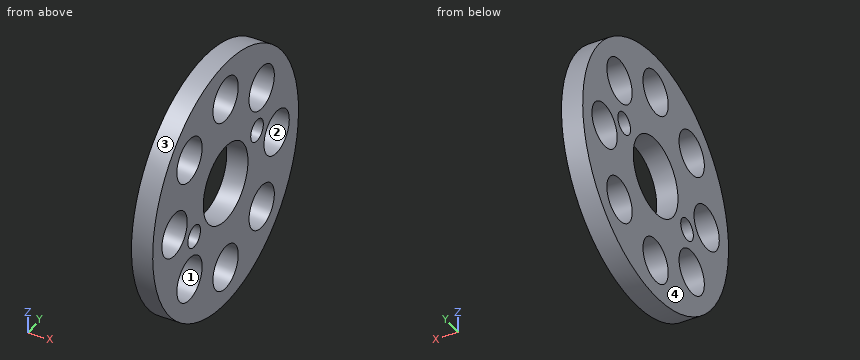
```python
from build123d import *

# Parameters (mm, degrees)
AXIAL_PROFILE_MM_W     = 5
AXIAL_PROFILE_MM_H     = 20.8
AXIAL_HOLES_DEPTH      = 155.634051877
AXIAL_HOLES_DEPTH_BACK = 155.634051877
SKETCH2_R              = 5.2
SKETCH2_R_2            = 2.6


with BuildPart() as part:
    # Axial profile (mm) → Full revolution (revolve)
    with BuildSketch(Plane.XY, mode=Mode.PRIVATE) as full_revolution_sk:
        with Locations((146.2, 19.6)):
            Rectangle(AXIAL_PROFILE_MM_W, AXIAL_PROFILE_MM_H)
    revolve(full_revolution_sk.sketch.rotate(Axis((-110, 0, 0), (1, 0, 0)), 90), axis=Axis((-110, 0, 0), (1, 0, 0)))

    # Sketch2 → Axial holes (cut, two sides: drawn at the far end of the back side and taken through both)
    with BuildSketch(Plane(origin=(0, 0, 0), x_dir=(0, 0, -1), z_dir=(1, 0, 0)).offset(-AXIAL_HOLES_DEPTH_BACK)):
        with Locations((0, 21)):
            Circle(SKETCH2_R)
        with Locations((-14.849242405, 14.849242405)):
            Circle(SKETCH2_R)
        with Locations((-21, 0)):
            Circle(SKETCH2_R)
        with Locations((-14.849242405, -14.849242405)):
            Circle(SKETCH2_R)
        with Locations((0, -21)):
            Circle(SKETCH2_R)
        with Locations((14.849242405, -14.849242405)):
            Circle(SKETCH2_R)
        with Locations((21, 0)):
            Circle(SKETCH2_R)
        with Locations((14.849242405, 14.849242405)):
            Circle(SKETCH2_R)
        with Locations((-5.357568053, 12.934313455)):
            Circle(SKETCH2_R_2)
        with Locations((5.357568053, -12.934313455)):
            Circle(SKETCH2_R_2)
    extrude(amount=AXIAL_HOLES_DEPTH + AXIAL_HOLES_DEPTH_BACK, mode=Mode.SUBTRACT)


solid = part.part
```
The model under review builds one solid part; all positions refer to its coordinate system, in mm. Face numbers are marked on the shaded views. Coordinates: 2 decimals unless noted, no trailing zeros. Write each loop counter-clockwise with the first axis right and the second up, starting at its lowest first coordinate (ties: lowest second). Pieces come first, ordered by that corner, then holes. Notation, with made-up numbers: (50, -21) - (92, -21) arc R25 cw to (92, 11) - close; hole circle Ø4 at (83, 67.5). An arc over 180 degrees is marked (long way). Answer in a Markdown table with one row per item. Add a question column.
Q1. Clearance check with flat-ended pins moving along their axes: pin 1 (4 mm diameter, centred on y = -12.93, z = -5.36, fed in from -X); pin 2 (1 mm diameter, centred on x = 145.5, y = -15.5, fed in from -Z); pin 3 (2 mm diameter, centred on x = 148, z = 3, fed in from +Y). State where each tip first meets the part, or that it passes through.
Q2. Consider section B-B on y = 19. Give the boundary of the cut face in (x, z), then the cut area to 3 significant figures.
Q3. Consider section C-C on z = -11.5. Give the boundary of the cut face in (x, y), then the cut area to 3 significant figures.
Q4. Consider section A-A on z = 0. Give the boundary of the cut face in (x, y), then the cut area to 3 significant figures.
Q5. To check wall thickness, follow line 1 along Y through (x, z) = (145, 0); line 2 along Z through (x, y) = (145, 0.5); line 3 along Y through (x, z) = (146.55, 10.5). State the ranges of each line that lie inside material, in increasing order. Write a range as from..to.
Q6. Consider section D-D on z = 21. Give the boundary of the cut face in (x, y), then the cut area to 3 significant figures.
Q7. Draft analysis for pull direction Y (two halves, no side actions). For the marked faces 1, 2, 3 and 4, state which applies: +Y half, -Y half, draft (parallel to the pull), parting line (faces both ways), or undercut.
Answers below:
| question | item | result |
|---|---|---|
| 1 | pin 1 | through |
| 1 | pin 2 | z = -25.98 |
| 1 | pin 3 | y = 29.93 |
| 2 | outline | (143.7, -23.22) - (148.7, -23.22) - (148.7, -17.98) - (143.7, -17.98) - close; (143.7, -11.72) - (148.7, -11.72) - (148.7, -4.8) - (143.7, -4.8) - close; (143.7, 4.8) - (148.7, 4.8) - (148.7, 11.72) - (143.7, 11.72) - close; (143.7, 17.98) - (148.7, 17.98) - (148.7, 23.22) - (143.7, 23.22) - close |
| 2 | area | 122 mm² |
| 3 | outline | (143.7, -27.71) - (148.7, -27.71) - (148.7, -18.83) - (143.7, -18.83) - close; (143.7, -10.87) - (148.7, -10.87) - (148.7, 10.87) - (143.7, 10.87) - close; (143.7, 18.83) - (148.7, 18.83) - (148.7, 27.71) - (143.7, 27.71) - close |
| 3 | area | 198 mm² |
| 4 | outline | (143.7, -30) - (148.7, -30) - (148.7, -26.2) - (143.7, -26.2) - close; (143.7, -15.8) - (148.7, -15.8) - (148.7, -9.2) - (143.7, -9.2) - close; (143.7, 9.2) - (148.7, 9.2) - (148.7, 15.8) - (143.7, 15.8) - close; (143.7, 26.2) - (148.7, 26.2) - (148.7, 30) - (143.7, 30) - close |
| 4 | area | 104 mm² |
| 5 | line 1 | -30..-26.2, -15.8..-9.2, 9.2..15.8, 26.2..30 |
| 5 | line 2 | -30..-26.18, -15.82..-9.19, 9.19..15.82, 26.18..30 |
| 5 | line 3 | -28.1..-17.7, -12..12, 17.7..28.1 |
| 6 | outline | (143.7, -21.42) - (148.7, -21.42) - (148.7, -5.2) - (143.7, -5.2) - close; (143.7, 5.2) - (148.7, 5.2) - (148.7, 21.42) - (143.7, 21.42) - close |
| 6 | area | 162 mm² |
| 7 | face 1 | undercut |
| 7 | face 2 | undercut |
| 7 | face 3 | parting line |
| 7 | face 4 | draft |
